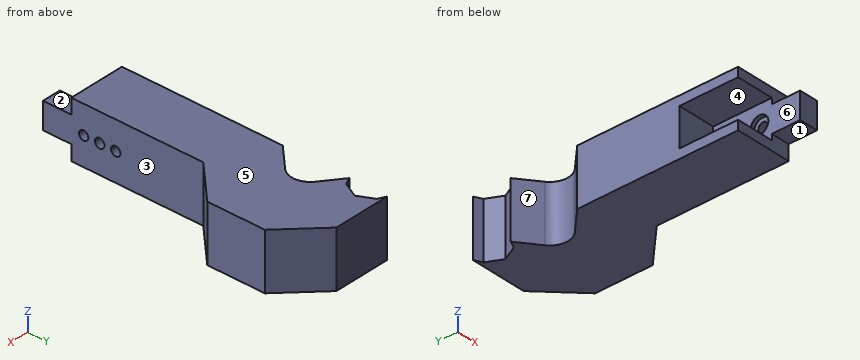
Autodesk Inventor part; units mm, degrees
ref_plane "YZ Plane" through (0, 0, 0) normal (1, 0, 0) x (0, 1, 0)
ref_plane "XZ Plane" through (0, 0, 0) normal (0, 1, 0) x (-1, 0, 0)
ref_plane "XY Plane" through (0, 0, 0) normal (0, 0, 1) x (1, 0, 0)
sketch "Sketch1" plane through (0, 0, 0) normal (0, 0, 1) x (1, 0, 0)
  line L0 (0, 0) -> (25, 0)
  line L1 (25, 0) -> (25, 40)
  line L2 (25, 40) -> (0, 40)
  line L3 (0, 40) -> (0, 0)
  dimension "d1" = 25
  dimension "d2" = 40
  dimension "d3" = 25
extrude "Extrusion1" add sketch "Sketch1" against normal blind 30
sketch "Sketch2" plane through (25, 0, 0) normal (1, 0, 0) x (0, 0, -1)
  line L0 (0, 0) -> (30, 0)
  circle A0 centre (15, 6.56) radius 2.46
extrude "Extrusion2" cut sketch "Sketch2" against normal blind 30
sketch "Sketch3" plane through (0, 0, 0) normal (-1, 0, 0) x (0, 0, 1)
  line L0 (0, 0) -> (-30, 0)
  line L1 (-25.05, 0) -> (-4.95, 0)
  line L2 (-4.95, 0) -> (-4.95, 33.12)
  line L3 (-4.95, 33.12) -> (-25.05, 33.12)
  line L4 (-25.05, 33.12) -> (-25.05, 0)
  dimension "d11" = 20.1
extrude "Extrusion3" cut sketch "Sketch3" against normal blind 20
sketch "Sketch4" plane through (0, 0, 0) normal (0, -1, 0) x (1, 0, 0)
  line L0 (20, -4.95) -> (20, -25.05)
  line L1 (20, -15) -> (25, -15)
  line L2 (25, 0) -> (25, -30)
  line L3 (20, -8.025) -> (25, -8.025)
  line L4 (25, -8.025) -> (25, -21.975)
  line L5 (25, -21.975) -> (20, -21.975)
  line L6 (20, -21.975) -> (20, -8.025)
  line L7 (20, -8.025) -> (25, -21.975) construction
  line L8 (25, -8.025) -> (20, -21.975) construction
  line L9 (25, -12.54) -> (25, -17.46)
  point P0 (0, 0)
  point P1 (22.5, -15)
  dimension "d14" = 13.95
extrude "Extrusion4" add sketch "Sketch4" along normal blind 15
sketch "Sketch5" plane through (20, 0, 0) normal (-1, 0, 0) x (0, 0, 1)
  circle A0 centre (-15, 6.56) radius 2.46
  circle A1 centre (-15, 6.56) radius 4.7025
  circle A2 centre (-15, 6.56) radius 2.46
  circle A3 centre (-15, 6.56) radius 2.46
  point P0 (0, 0)
  dimension "d17" = 9.405
extrude "Extrusion5" cut sketch "Sketch5" against normal blind 2.1
sketch "Sketch6" plane through (25, 0, 0) normal (1, 0, 0) x (0, 0, -1)
  circle A0 centre (15, 6.56) radius 4.7025
  line L0 (15, 6.56) -> (15, 23.56)
  circle A1 centre (15, 23.56) radius 2.46
  point P0 (0, 0)
  dimension "d20" = 17
  dimension "d21" = 4.92
extrude "Extrusion6" cut sketch "Sketch6" against normal blind 10 contours A1
sketch "Sketch7" plane through (20, 0, 0) normal (-1, 0, 0) x (0, 0, 1)
  circle A0 centre (-15, 23.56) radius 2.46
  circle A1 centre (-15, 23.56) radius 4.7025
  point P0 (0, 0)
  dimension "d24" = 9.405
extrude "Extrusion7" cut sketch "Sketch7" against normal blind 2.1
sketch "Sketch9" plane through (25, 0, 0) normal (1, 0, 0) x (0, 0, -1)
  circle A0 centre (15, 6.56) radius 2.46
  circle A1 centre (15, 6.56) radius 2.46
  circle A2 centre (15, 23.56) radius 2.46
  circle A3 centre (15, 23.56) radius 2.46
  line L0 (30, 40) -> (30, 0)
  line L1 (30, 0) -> (30, 40)
  line L2 (30, 40) -> (0, 40)
  line L3 (0, 40) -> (0, 0)
  line L4 (0, 0) -> (8.025, 0)
  line L5 (21.975, 0) -> (21.975, -15)
  line L6 (21.975, -15) -> (8.025, -15)
  line L7 (8.025, -15) -> (8.025, 0)
  line L8 (0, 0) -> (8.025, 0)
  line L9 (21.975, 0) -> (30, 0)
extrude "Extrusion8" add sketch "Sketch9" along normal blind 5
sketch "Sketch10" plane through (0, 40, 0) normal (0, 1, 0) x (1, 0, 0)
  line L0 (0, 30) -> (30, 30)
  line L1 (30, 0) -> (0, 0)
  line L2 (0, 30) -> (30, 30)
  line L3 (30, 30) -> (30, 0)
  line L4 (30, 0) -> (0, 0)
  line L5 (0, 0) -> (0, 30)
extrude "Extrusion9" add sketch "Sketch10" along normal blind 30
sketch "Sketch12" plane through (30, 0, 0) normal (1, 0, 0) x (0, 0, -1)
  circle A0 centre (15, 6.56) radius 2.46
  line L0 (15, 6.56) -> (15, 15.06)
  circle A1 centre (15, 15.06) radius 2.525
  point P0 (0, 0)
  dimension "d31" = 8.5
  dimension "d33" = 5.05
extrude "Extrusion10" cut sketch "Sketch12" against normal blind 30 contours A1
sketch "Sketch15" plane through (0, 0, -25.05) normal (-1, 0, 0) x (0, 0, 1)
  line L0 (0, 33.12) -> (20.1, 33.12)
  line L1 (20.1, 33.12) -> (20.1, 0)
  line L2 (0, 33.12) -> (20.1, 33.12)
  line L3 (20.1, 33.12) -> (20.1, 31.1)
  line L4 (20.1, 31.1) -> (0, 31.1)
  line L5 (0, 31.1) -> (0, 33.12)
  point P0 (25.05, 0)
  dimension "d57" = 2.02
extrude "Extrusion13" add sketch "Sketch15" against normal blind 20
sketch "Sketch17" plane through (0, 0, 0) normal (0, 0, 1) x (1, 0, 0)
  line L0 (0, 70) -> (30, 70)
  line L1 (30, 70) -> (50.0622, 90.0622)
  line L2 (30, 70) -> (80, 70) construction
  line L3 (11.9522, 97.2454) -> (0, 85.2932)
  line L4 (0, 70) -> (0, 85.2932)
  line L5 (0, 70) -> (0, 0)
  line L6 (0, 70) -> (30, 70)
  line L7 (10.923, 112.2849) -> (0, 120.567)
  line L8 (50.0622, 105.3553) -> (50.0622, 120.567)
  line L9 (50.0622, 105.3553) -> (50.0622, 90.0622)
  arc A0 (11.9522, 97.2454) -> (10.923, 112.2849) centre (4.8811, 104.3165) ccw
  line L10 (4, 138.567) -> (0, 140.567)
  line L11 (4, 122.567) -> (0, 120.567)
  line L12 (4, 122.567) -> (8, 130.567)
  line L13 (4, 138.567) -> (8, 130.567)
  line L14 (0, 140.567) -> (30, 140.567)
  line L15 (30, 140.567) -> (50.0622, 120.567)
  dimension "d61" = 45
  dimension "d62" = 32.0271
  dimension "d72" = 10
extrude "Extrusion14" add sketch "Sketch17" against normal blind 30
properties part number "rec_c_16mm_x_30mm"
Verification items for the finished model (mm, model axes). Face numbers are marked on the shaded views. A direction names the side the tool comes from. Coordinates: 2 decimals unless noted, no trailing zeros. Loops run counter-clockwise (first coordinate to the right, second up) from the corner with the lowest first, then second, coordinate; pieces in that order, holes last. Notation, with made-up numbers: (70.25, 57) -> (87.25, 57) arc R11 ccw to (87.25, 69) -> close; hole circle Ø5 at (18.5, -30.75). An arc over 180 degrees is marked (long way). Put each result on its own line as item: value.
1. Tool access check on the marked faces 5, 6 and 7. Record the directions out of +Z, -Z, +X, -X, +Y, -Y that give a thin tool (end or side, any length) a straight path to the whole face; none if there is none.
Result set:
face 5: +Z, +X, -X, +Y, -Y
face 6: -X, -Y
face 7: +Z, -Z, -X
2. Section check B-B, the plane z = -2.75. Record the boundary of the cut face in (x, y).
Result set:
outline: (0, 0) -> (30, 0) -> (30, 70) -> (50.06, 90.06) -> (50.06, 120.57) -> (30, 140.57) -> (0, 140.57) -> (4, 138.57) -> (8, 130.57) -> (4, 122.57) -> (0, 120.57) -> (10.92, 112.28) arc R10 cw to (11.95, 97.25) -> (0, 85.29) -> close
3. Section check A-A, the plane y = 15.06. Record the boundary of the cut face in (x, z) (3 decimals).
Result set:
outline: (0, -30) -> (30, -30) -> (30, -17.525) -> (20, -17.525) -> (20, -25.05) -> (0, -25.05) -> close; (0, -4.95) -> (20, -4.95) -> (20, -12.475) -> (30, -12.475) -> (30, 0) -> (0, 0) -> close
4. Gauge pin test, flat ends, axial feed: P1, Ø4.5, axis at y = 5.5, z = -13, coming from the -X side; P2, Ø4.5, axis at y = 23.56, z = -15, coming from the +X side; P3, Ø4, axis at x = 19.5, z = -3.5, coming from the -Y side; P4, Ø8.5, axis at y = 23.56, z = -15, coming from the +X side. Record the tip position at first contact, or that the pin passes through.
Result set:
P1: stops at x = 22.1
P2: passes through
P3: stops at y = 0
P4: stops at x = 30
5. Section check C-C, the plane z = -15. Give the number of separate pieces and of enclosed holes in the cut face, then the cut area to 3 significant figures.
Result set:
separate pieces: 4
enclosed holes: 0
area: 4,160 mm^2
6. Mould release check, pull along Z, two halves, no side actions. Record for the marked faces 1, 2, 3 and 4: pulls with the +Z half, pulls with the -Z half, needs draft (parallel to the pull), parting line crosses it, or undercut.
Result set:
face 1: pulls with the -Z half
face 2: pulls with the +Z half
face 3: needs draft
face 4: undercut
7. Section check D-D, the plane y = -4. Record the boundary of the cut face in (x, z) (3 decimals).
Result set:
outline: (20, -21.975) -> (30, -21.975) -> (30, -8.025) -> (20, -8.025) -> close
8. Thickness scan on line 1 (Y direction, x = 26.25, z = -15) (3 decimals); line 2 (Z direction, x = 21, y = 6); line 3 (Z direction, x = 7, y = 1.5). Record the ranges inside material, lowest first.
Result set:
line 1: y = -15 to 4.1, 9.02 to 12.535, 17.585 to 21.1, 26.02 to 140.567
line 2: z = -30 to -19.67, -10.33 to 0
line 3: z = -30 to -25.05, -4.95 to 0
